Build history of the part. All positions in model axes, mm. A direction names the side the tool comes from. Round coordinates to 2 decimals unless told otherwise and drop trailing zeros. Loops run counter-clockwise (first coordinate to the right, second up) from the corner with the lowest first, then second, coordinate; pieces in that order, holes last. Notation, with made-up numbers: (-15, 23.5) - (19, 23.5) arc R11 ccw to (19, 33.5) - close; hole circle Ø9 at (6.25, 76). An arc over 180 degrees is marked (long way). One line per question, with ' | ' between items. Start each with the question number.
from build123d import *

# Parameters (mm, degrees)
F0_W           = 304.8
F0_H           = 304.8
F1_DEPTH       = 4.2333333333
F2_R           = 14.097
F2_R_2         = 10.287
F3_DEPTH       = 6.35
F4_W           = 39.3954
F4_H           = 39.3954
F5_DEPTH       = 3.175
F6_W           = 39.3954
F6_H           = 76.2
F7_DEPTH       = 3.175
F9_R           = 1.905
F10_DEPTH      = 129.414
F10_DEPTH_BACK = 86.36


with BuildPart() as f1:
    # F0 (on Top) → F1 (new body)
    with BuildSketch(Plane.XY):
        Rectangle(F0_W, F0_H)
    extrude(amount=F1_DEPTH)

    # F2 (on face) → F3 (join)
    with BuildSketch(Plane.XY.offset(4.2333333333)):
        with Locations((127, 0)):
            Circle(F2_R)
        with Locations((127, 0)):
            Circle(F2_R_2, mode=Mode.SUBTRACT)
    extrude(amount=F3_DEPTH)

    # F4 (on face) → F5 (join)
    with BuildSketch(Plane.XY.offset(4.2333333333)):
        with Locations((127, 42.6847)):
            Rectangle(F4_W, F4_H)
        with Locations((127, -42.6847)):
            Rectangle(F4_W, F4_H)
    extrude(amount=F5_DEPTH)

    # F6 (on face) → F7 (join)
    with BuildSketch(Plane.XZ.offset(-22.987)):
        with Locations((127, 42.3333333333)):
            Rectangle(F6_W, F6_H)
        with BuildLine():
            ThreePointArc((146.6977, 80.4333333333), (127, 100.1310333333), (107.3023, 80.4333333333))
            Line((107.3023, 80.4333333333), (146.6977, 80.4333333333))
        make_face()
    extrude(amount=-F7_DEPTH)

    # F8: F1 across plane


with BuildPart() as f1_1:
    add(f1.part)
    add(f1.part.mirror(Plane.XZ))

    # F9 (on face) → F10 (cut, two sides)
    with BuildSketch(Plane.XZ.offset(-22.987)) as f10_sk:
        with Locations((127, 42.3333333333)):
            Circle(F9_R)
        with Locations((127, 80.4333333333)):
            Circle(F9_R)
    extrude(amount=-F10_DEPTH, mode=Mode.SUBTRACT)
    extrude(f10_sk.sketch, amount=F10_DEPTH_BACK, mode=Mode.SUBTRACT)


solid = f1_1.part
1) Saw through at C-C on z = 90. Write the cut outline in (x, y).
2) Saw through at B-B on y = -54.5. Write the cut outline in (x, z), and give its area (3 significant figures).
3) Drop flat-ended pins along their axis: pin 1 (19.5 mm diameter, centred on x = 132.5, z = 67, fed in from -Y); pin 2 (3 mm diameter, centred on x = -10.5, y = -59.5, fed in from +Z); pin 3 (3.5 mm diameter, centred on x = 127, z = 80.43, fed in from +Y); pin 4 (8.5 mm diameter, centred on x = 121, y = 1.5, fed in from +Z). Give the stop position or say it passes through.
4) Saw through at A-A on z = 52. Write the cut outline in (x, y).
5) Saw through at D-D on y = 0. Write the cut outline in (x, z).
6) Two-plate mould, pull along Y, no slides. Class faces 5 (the flat face through (127, -26.162, 54)), 6 (the flat face through (127, 45, 7.408)), 7 (the cylindrical face through (116.723, 0.452, 7.364)), 8 (the flat face through (127, 26.162, 54)): +Y half, -Y half, draft (parallel to the pull), parting line (faces both ways), or undercut.
7) Wall check: line 1 (Z direction, x = 127, y = 25); line 2 (Y direction, x = 127, z = 6); line 3 (X direction, y = 24, z = 69.5). Give the ranges that are in metal, low to high. Write a range as [from, to].
8) Tool access for faces 1 (the flat face through (146.698, 25, 31)), 2 (the flat face through (107.302, -25, 31)), 3 (the cylindrical face through (140.446, 4.234, 7.364)), 4 (the flat face through (127, 22.987, 52)): list every direction of +Z, -Z, +X, -X, +Y, -Y with a clear straight run to the whole face (end or side of a thin tool).
Answer key:
1) outline: (109.78, -26.16) - (144.22, -26.16) - (144.22, -22.99) - (109.78, -22.99) - close; (109.78, 22.99) - (144.22, 22.99) - (144.22, 26.16) - (109.78, 26.16) - close
2) outline: (-152.4, 0) - (152.4, 0) - (152.4, 4.23) - (146.7, 4.23) - (146.7, 7.41) - (107.3, 7.41) - (107.3, 4.23) - (-152.4, 4.23) - close | area: 1,420 mm²
3) pin 1: y = -26.16 | pin 2: z = 4.23 | pin 3: through | pin 4: z = 10.58
4) outline: (107.3, -26.16) - (146.7, -26.16) - (146.7, -22.99) - (107.3, -22.99) - close; (107.3, 22.99) - (146.7, 22.99) - (146.7, 26.16) - (107.3, 26.16) - close
5) outline: (-152.4, 0) - (152.4, 0) - (152.4, 4.23) - (141.1, 4.23) - (141.1, 10.58) - (137.29, 10.58) - (137.29, 4.23) - (116.71, 4.23) - (116.71, 10.58) - (112.9, 10.58) - (112.9, 4.23) - (-152.4, 4.23) - close
6) face 5: -Y half | face 6: draft | face 7: undercut | face 8: +Y half
7) line 1: [0, 40.43], [44.24, 78.53], [82.34, 100.13] | line 2: [-62.38, -22.99], [-14.1, -10.29], [10.29, 14.1], [22.99, 62.38] | line 3: [107.3, 146.7]
8) face 1: +Z, +X, +Y, -Y | face 2: +Z, -X, +Y, -Y | face 3: +Z | face 4: +Z, +X, -X
